```python
from build123d import *

# Parameters (mm, degrees)
BOSS_EXTRUDE1_DEPTH = 100
SHELL1_T            = -5
CHAMFER1_SIZE       = 10
CHAMFER2_SIZE       = 10
FILLET2_R           = 10
CUT_EXTRUDE1_DEPTH  = 250
BOSS_EXTRUDE5_DEPTH = 60
SKETCH8_W           = 41
SKETCH8_H           = 21
BOSS_EXTRUDE6_DEPTH = 31
SKETCH12_W          = 51
SKETCH12_H          = 45
BOSS_EXTRUDE7_DEPTH = 50
SKETCH26_R          = 19
CUT_EXTRUDE2_DEPTH  = 29
SKETCH28_R          = 17.75
CUT_EXTRUDE3_DEPTH  = 22
BOSS_EXTRUDE8_DEPTH = 60
SKETCH30_W          = 10.5
SKETCH30_H          = 9
CUT_EXTRUDE4_DEPTH  = 29
FILLET4_R           = 10
SKETCH32_W          = 15
SKETCH32_H          = 10
CUT_EXTRUDE7_DEPTH  = 10
CUT_EXTRUDE8_DEPTH  = 10
SKETCH37_W          = 177.863308591
SKETCH37_H          = 31
CUT_EXTRUDE10_DEPTH = 84
FILLET11_R          = 10


with BuildPart() as part:
    # Sketch2 → Boss-Extrude1 (new body)
    with BuildSketch(Plane(origin=(0, 0, 0), x_dir=(1, 0, 0), z_dir=(0, 1, 0))):
        Polygon((-11.910210202, -80), (-11.910210202, 80), (-191.910210202, 80), (-266.188345473, 50.288745892), (-266.188345473, -50.288745892), (-191.910210202, -80), align=None)
    extrude(amount=BOSS_EXTRUDE1_DEPTH)

    # Shell1
    shell1_openings = [part.faces().sort_by_distance(p)[0] for p in [
        (-133.177254811, 100, 0),
    ]]
    offset(amount=SHELL1_T, openings=shell1_openings, kind=Kind.INTERSECTION)

    # Chamfer1
    # the kernel refuses this chamfer: 10 mm, written as the material it takes off along each edge
    with BuildSketch(Plane(origin=(-11.910210202, 100, 105.71682988), x_dir=(0.027495876610586317, -0.9996219169112968, 0), z_dir=(0, 0, -1))) as chamfer1_piece_1:
        Polygon((CHAMFER1_SIZE * 0.999621916911, CHAMFER1_SIZE * 0.0274958766106), (-CHAMFER1_SIZE * 0.0274958766106, CHAMFER1_SIZE * 0.999621916911), (0, 0), align=None)
    extrude(amount=211.433659759, mode=Mode.SUBTRACT)

    # Chamfer2
    # the kernel refuses this chamfer: 10 mm, written as the material it takes off along each edge
    with BuildSketch(Plane(origin=(-266.188345473, 100, -76.005575771), x_dir=(-0.0274958766105877, -0.9996219169112968, 0), z_dir=(0, 0, 1))) as chamfer2_piece_1:
        Polygon((CHAMFER2_SIZE * 0.999621916911, CHAMFER2_SIZE * 0.0274958766106), (-CHAMFER2_SIZE * 0.0274958766106, CHAMFER2_SIZE * 0.999621916911), (0, 0), align=None)
    extrude(amount=152.011151543, mode=Mode.SUBTRACT)

    # Fillet2
    fillet2_edges = [part.edges().sort_by_distance(p)[0] for p in [
        (-11.910210202, 0, 0),
        (-101.910210202, 0, 80),
        (-229.049277838, 0, 65.144372946),
        (-266.188345473, 0, 0),
        (-229.049277838, 0, -65.144372946),
        (-101.910210202, 0, -80),
    ]]
    fillet(fillet2_edges, radius=FILLET2_R)

    # Sketch3 → Cut-Extrude1 (cut)
    with BuildSketch(Plane.XY.offset(80)):
        Polygon((-191.910210202, 100), (-266.188345473, 65.891137916), (-266.188345473, 100), align=None)
    extrude(amount=-CUT_EXTRUDE1_DEPTH, mode=Mode.SUBTRACT)

    # Sketch4 → Boss-Extrude5 (add)
    with BuildSketch(Plane(origin=(0, 5, 0), x_dir=(1, 0, 0), z_dir=(0, 1, 0))):
        Polygon((-215.188345473, -15.5), (-444.051654064, -15.5), (-444.051654064, 15.5), (-261.610116413, 15.5), (-215.188345473, 15.5), align=None)
        Polygon((-261.188345473, 10.5), (-220.188345473, 10.5), (-220.188345473, -10.5), (-384.777774205, -10.5), (-384.777774205, 9.502386243), align=None, mode=Mode.SUBTRACT)
    extrude(amount=BOSS_EXTRUDE5_DEPTH)

    # Sketch8 → Boss-Extrude6 (add)
    with BuildSketch(Plane(origin=(0, 5, 0), x_dir=(1, 0, 0), z_dir=(0, 1, 0))):
        with Locations((-240.688345473, 0)):
            Rectangle(SKETCH8_W, SKETCH8_H)
    extrude(amount=BOSS_EXTRUDE6_DEPTH)

    # Sketch12 → Boss-Extrude7 (add)
    with BuildSketch(Plane(origin=(-11.910210202, 0, 0), x_dir=(0, 0, -1), z_dir=(1, 0, 0))):
        with Locations((-54.5, 50)):
            Rectangle(SKETCH12_W, SKETCH12_H)
    boss_extrude7 = extrude(amount=BOSS_EXTRUDE7_DEPTH)

    # Sketch26 → Cut-Extrude2 (cut)
    with BuildSketch(Plane.XY.offset(80)):
        with Locations((13.089789798, 50)):
            Circle(SKETCH26_R)
    cut_extrude2 = extrude(amount=-CUT_EXTRUDE2_DEPTH, mode=Mode.SUBTRACT)

    # Sketch28 → Cut-Extrude3 (cut)
    with BuildSketch(Plane.XY.offset(51)):
        with Locations((13.089789798, 50)):
            Circle(SKETCH28_R)
    cut_extrude3 = extrude(amount=-CUT_EXTRUDE3_DEPTH, mode=Mode.SUBTRACT)

    # Mirror1: Boss-Extrude7, Cut-Extrude2, Cut-Extrude3 across plane
    add(boss_extrude7.mirror(Plane.XY))
    add(cut_extrude2.mirror(Plane.XY), mode=Mode.SUBTRACT)
    add(cut_extrude3.mirror(Plane.XY), mode=Mode.SUBTRACT)

    # Sketch29 → Boss-Extrude8 (add)
    with BuildSketch(Plane(origin=(0, 65, 0), x_dir=(1, 0, 0), z_dir=(0, 1, 0))):
        Polygon((-261.188345473, 20.5), (-210.188345473, 20.5), (-210.188345473, -20.5), (-261.188345473, -20.5), (-261.188345473, -15.5), (-215.188345473, -15.5), (-215.188345473, 15.5), (-261.188345473, 15.5), align=None)
    extrude(amount=-BOSS_EXTRUDE8_DEPTH)

    # Sketch30 → Cut-Extrude4 (cut)
    with BuildSketch(Plane(origin=(0, 65, 0), x_dir=(1, 0, 0), z_dir=(0, 1, 0))):
        with Locations((-215.438345473, 0)):
            Rectangle(SKETCH30_W, SKETCH30_H)
    extrude(amount=-CUT_EXTRUDE4_DEPTH, mode=Mode.SUBTRACT)

    # Fillet4
    fillet4_edges = [part.edges().sort_by_distance(p)[0] for p in [
        (38.089789798, 72.5, 54.5),
        (38.089789798, 27.5, 54.5),
        (38.089789798, 27.5, -54.5),
        (38.089789798, 72.5, -54.5),
    ]]
    fillet(fillet4_edges, radius=FILLET4_R)

    # Sketch32 → Cut-Extrude7 (cut)
    with BuildSketch(Plane(origin=(-11.910210202, 0, 0), x_dir=(0, 0, -1), z_dir=(1, 0, 0))):
        with Locations((0, 50)):
            Rectangle(SKETCH32_W, SKETCH32_H)
    extrude(amount=-CUT_EXTRUDE7_DEPTH, mode=Mode.SUBTRACT)

    # Sketch34 → Cut-Extrude8 (cut)
    with BuildSketch(Plane(origin=(0, 0, -80), x_dir=(-1, 0, 0), z_dir=(0, 0, -1))):
        with BuildLine():
            Line((175.162205164, 97.108614193), (180.250510852, 97.108614193))
            ThreePointArc((180.250510852, 97.108614193), (181.878966661, 95.480158384), (180.250510852, 93.851702575))
            Line((180.250510852, 93.851702575), (175.162205164, 93.851702575))
            ThreePointArc((175.162205164, 93.851702575), (173.533749356, 95.480158384), (175.162205164, 97.108614193))
        make_face()
        with BuildLine():
            Line((160.318525442, 97.108614193), (165.401872055, 97.108614193))
            ThreePointArc((165.401872055, 97.108614193), (167.030327863, 95.480158384), (165.401872055, 93.851702575))
            Line((165.401872055, 93.851702575), (160.318525442, 93.851702575))
            ThreePointArc((160.318525442, 93.851702575), (158.690069633, 95.480158384), (160.318525442, 97.108614193))
        make_face()
        with BuildLine():
            Line((175.160903312, 17.203664766), (180.240903312, 17.203664766))
            ThreePointArc((180.240903312, 17.203664766), (181.865903312, 15.578664766), (180.240903312, 13.953664766))
            Line((180.240903312, 13.953664766), (175.160903312, 13.953664766))
            ThreePointArc((175.160903312, 13.953664766), (173.535903312, 15.578664766), (175.160903312, 17.203664766))
        make_face()
        with BuildLine():
            Line((160.324224815, 17.203664766), (165.404224815, 17.203664766))
            ThreePointArc((165.404224815, 17.203664766), (167.029224815, 15.578664766), (165.404224815, 13.953664766))
            Line((165.404224815, 13.953664766), (160.324224815, 13.953664766))
            ThreePointArc((160.324224815, 13.953664766), (158.699224815, 15.578664766), (160.324224815, 17.203664766))
        make_face()
    cut_extrude8 = extrude(amount=-CUT_EXTRUDE8_DEPTH, mode=Mode.SUBTRACT)

    # Mirror2: Cut-Extrude8 across plane
    add(cut_extrude8.mirror(Plane.XY), mode=Mode.SUBTRACT)

    # Sketch37 → Cut-Extrude10 (cut)
    with BuildSketch(Plane(origin=(0, 65, 0), x_dir=(1, 0, 0), z_dir=(0, 1, 0))):
        with Locations((-355.119999769, 0)):
            Rectangle(SKETCH37_W, SKETCH37_H)
    extrude(amount=-CUT_EXTRUDE10_DEPTH, mode=Mode.SUBTRACT)

    # Fillet11
    # the kernel refuses this fillet: 10 mm, written as the material it takes off along each edge
    with BuildSketch(Plane(origin=(-266.188345473, 5, 28), x_dir=(0, 1, 0), z_dir=(0, 0, -1))) as fillet11_piece_1:
        with BuildLine():
            CenterArc((5, 10), FILLET11_R, 240, 30)
            Line((0, 1.339745962), (-0.1, 1.166540881))
            ThreePointArc((-0.1, 1.166540881), (-0.2, 0.669872981), (-0.2, 0))
            Line((-0.2, 0), (0, -0.2))
            Line((0, -0.2), (5, -0.2))
            Line((5, -0.2), (5, 0))
        make_face()
    extrude(amount=30, mode=Mode.SUBTRACT)
    with BuildSketch(Plane(origin=(-266.188345473, 5, 2.040359995), x_dir=(0, 1, 0), z_dir=(0, 0, -1))) as fillet11_piece_2:
        with BuildLine():
            CenterArc((5, 10), FILLET11_R, 240, 30)
            Line((0, 1.339745962), (-0.1, 1.166540881))
            ThreePointArc((-0.1, 1.166540881), (-0.2, 0.669872981), (-0.2, 0))
            Line((-0.2, 0), (0, -0.2))
            Line((0, -0.2), (5, -0.2))
            Line((5, -0.2), (5, 0))
        make_face()
    extrude(amount=30.040359995, mode=Mode.SUBTRACT)


solid = part.part
```
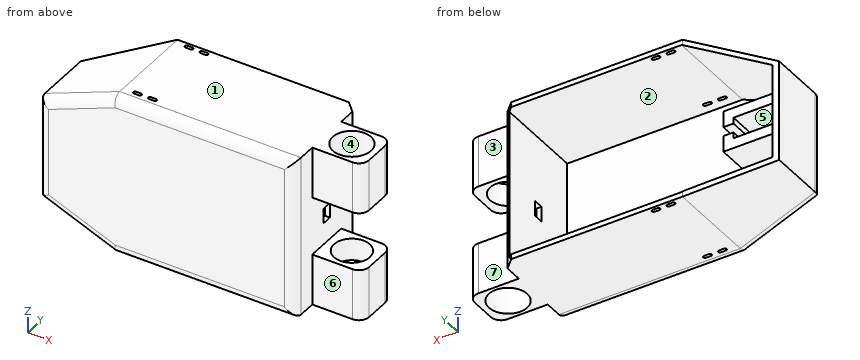
Verification items for the finished model (mm, model axes). Face numbers are marked on the shaded views. A direction names the side the tool comes from. Coordinates: 2 decimals unless noted, no trailing zeros. Loops run counter-clockwise (first coordinate to the right, second up) from the corner with the lowest first, then second, coordinate; pieces in that order, holes last. Notation, with made-up numbers: (83, -17) - (112, -17) arc R22 cw to (112, 4) - close; hole circle Ø8 at (45, -24). An arc over 180 degrees is marked (long way). Put each result on its own line as item: value.
Item 1: Section check C-C (y = 50). Give the number of separate pieces and of enclosed holes in the cut face, then the cut area to 3 significant figures.
Conclusion:
separate pieces: 3
enclosed holes: 0
area: 6,210 mm2
Item 2: Section check A-A (x = -92). Enter the section's corners in (y, z).
Conclusion:
outline: (0, -70) arc R10 ccw to (10, -80) - (100, -80) - (100, -75) - (5, -75) - (5, 75) - (100, 75) - (100, 80) - (10, 80) arc R10 ccw to (0, 70) - close
Item 3: Section check B-B (z = -34). Enter the section's corners in (x, y).
Conclusion:
outline: (-266.19, 10) arc R10 ccw to (-256.19, 0) - (-21.91, 0) arc R10 ccw to (-11.91, 10) - (-11.91, 27.5) - (28.09, 27.5) arc R10 ccw to (38.09, 37.5) - (38.09, 62.5) arc R10 ccw to (28.09, 72.5) - (-11.91, 72.5) - (-11.91, 90) - (-16.91, 95) - (-16.91, 5) - (-261.19, 5) - (-261.19, 68.19) - (-266.19, 65.89) - close; hole circle Ø35.5 at (13.09, 50)
Item 4: Set-up check for the marked faces 4, 5, 6 and 7: record each of +Z, -Z, +X, -X, +Y, -Y from which the full face is reachable in a straight line by a thin tool's end or side.
Conclusion:
face 4: +Z
face 5: +Y
face 6: +Z, -Z, +X, -Y
face 7: +Z, -Z, +X, +Y
Item 5: Gauge pin test, flat ends, axial feed: pin 1 Ø2 at (x, z) = (-88, 48.5) entering from +Y; pin 2 Ø14.5 at (x, y) = (-246, 47.5) entering from +Z; pin 3 Ø20.5 at (y, z) = (26, 0) entering from +X; pin 4 Ø21.5 at (x, y) = (13.09, 50) entering from -Z. Record the tip position at first contact, or that the pin passes through.
Conclusion:
pin 1: stops at y = 5
pin 2: stops at z = 61.26
pin 3: stops at x = -11.91
pin 4: passes through
Item 6: Draft check along Z on the marked faces 1, 2 and 3. Enter one of: pulls with the +Z half, pulls with the -Z half, needs draft (parallel to the pull), parting line crosses it, or undercut.
Conclusion:
face 1: pulls with the +Z half
face 2: undercut
face 3: needs draft
Item 7: Scan lines: line 1 along Z through (x, y) = (-103, 48); line 2 along X through (y, z) = (38.5, 14); line 3 along Y through (x, z) = (13, 60). Record each from-to range of solid material in increasing order.
Conclusion:
line 1: z = -80 to -75, 75 to 80
line 2: x = -266.19 to -210.19, -16.91 to -11.91
line 3: y = 27.5 to 31, 69 to 72.5
